```python
from build123d import *

# Parameters (mm, degrees)
SKETCH1_R           = 11
SKETCH1_R_2         = 2
SKETCH1_R_3         = 5
BOSS_EXTRUDE2_DEPTH = 5
BOSS_EXTRUDE4_DEPTH = 5
SKETCH2_W           = 50
SKETCH2_H           = 5
BOSS_EXTRUDE7_DEPTH = 45
CUT_EXTRUDE1_REACH  = 64.081
SKETCH3_R           = 3
FILLET1_R           = 10


with BuildPart() as part:
    # Sketch1 → Boss-Extrude2 (new body)
    with BuildSketch(Plane.XY):
        Circle(SKETCH1_R)
        with Locations((-8, 0)):
            Circle(SKETCH1_R_2, mode=Mode.SUBTRACT)
        with Locations((0, -8)):
            Circle(SKETCH1_R_2, mode=Mode.SUBTRACT)
        with Locations((8, 0)):
            Circle(SKETCH1_R_2, mode=Mode.SUBTRACT)
        with Locations((0, 8)):
            Circle(SKETCH1_R_2, mode=Mode.SUBTRACT)
        Circle(SKETCH1_R_3, mode=Mode.SUBTRACT)
    extrude(amount=BOSS_EXTRUDE2_DEPTH)

    # Sketch1_9 → Boss-Extrude4 (add)
    with BuildSketch(Plane.XY):
        with BuildLine():
            Line((-25, 16), (-25, 11))
            Line((-25, 11), (-15, 11))
            Line((-15, 11), (-11, 0))
            ThreePointArc((-11, 0), (0, 11), (11, 0))
            Line((11, 0), (15, 11))
            Line((15, 11), (25, 11))
            Line((25, 11), (25, 16))
            Line((25, 16), (-25, 16))
        make_face()
    extrude(amount=BOSS_EXTRUDE4_DEPTH)

    # Sketch2 → Boss-Extrude7 (add)
    with BuildSketch(Plane.XY.offset(5)):
        with Locations((0, 13.5)):
            Rectangle(SKETCH2_W, SKETCH2_H)
    extrude(amount=BOSS_EXTRUDE7_DEPTH)

    # Sketch3 → Cut-Extrude1 (cut, up to next)
    with BuildSketch(Plane(origin=(0, 16, 0), x_dir=(1, 0, 0), z_dir=(0, 1, 0)), mode=Mode.PRIVATE) as cut_extrude1_sk1:
        with Locations(Location((10, -35, 0), (0, 0, 270))):
            Circle(SKETCH3_R)
    cut_extrude1_tool1 = extrude(cut_extrude1_sk1.sketch, amount=-CUT_EXTRUDE1_REACH, mode=Mode.PRIVATE) & part.part
    # Sketch3 → Cut-Extrude1 (cut, up to next)
    with BuildSketch(Plane(origin=(0, 16, 0), x_dir=(1, 0, 0), z_dir=(0, 1, 0)), mode=Mode.PRIVATE) as cut_extrude1_sk2:
        with Locations(Location((-10, -35, 0), (0, 0, 270))):
            Circle(SKETCH3_R)
    cut_extrude1_tool2 = extrude(cut_extrude1_sk2.sketch, amount=-CUT_EXTRUDE1_REACH, mode=Mode.PRIVATE) & part.part
    # Sketch3 → Cut-Extrude1 (cut, up to next)
    with BuildSketch(Plane(origin=(0, 16, 0), x_dir=(1, 0, 0), z_dir=(0, 1, 0)), mode=Mode.PRIVATE) as cut_extrude1_sk3:
        with Locations(Location((-10, -15, 0), (0, 0, 270))):
            Circle(SKETCH3_R)
    cut_extrude1_tool3 = extrude(cut_extrude1_sk3.sketch, amount=-CUT_EXTRUDE1_REACH, mode=Mode.PRIVATE) & part.part
    # Sketch3 → Cut-Extrude1 (cut, up to next)
    with BuildSketch(Plane(origin=(0, 16, 0), x_dir=(1, 0, 0), z_dir=(0, 1, 0)), mode=Mode.PRIVATE) as cut_extrude1_sk4:
        with Locations(Location((10, -15, 0), (0, 0, 270))):
            Circle(SKETCH3_R)
    cut_extrude1_tool4 = extrude(cut_extrude1_sk4.sketch, amount=-CUT_EXTRUDE1_REACH, mode=Mode.PRIVATE) & part.part
    add(cut_extrude1_tool1.solids().sort_by_distance((10, 16, 35))[0], mode=Mode.SUBTRACT)
    add(cut_extrude1_tool2.solids().sort_by_distance((-10, 16, 35))[0], mode=Mode.SUBTRACT)
    add(cut_extrude1_tool3.solids().sort_by_distance((-10, 16, 15))[0], mode=Mode.SUBTRACT)
    add(cut_extrude1_tool4.solids().sort_by_distance((10, 16, 15))[0], mode=Mode.SUBTRACT)

    # Fillet1
    fillet1_edges = [part.edges().sort_by_distance(p)[0] for p in [
        (25, 13.5, 0),
        (25, 13.5, 50),
        (-25, 13.5, 0),
        (-25, 13.5, 50),
    ]]
    fillet(fillet1_edges, radius=FILLET1_R)


solid = part.part
```
CAD build for the part. Positions are in the model's coordinates, mm. A direction names the side the tool comes from. Coordinates: 2 decimals unless noted, no trailing zeros. Order: outer loops, then holes, each group sorted by start corner. A loop starts at its lowest first (then second) coordinate and runs counter-clockwise, first axis right, second up. Notation, with made-up numbers: M 75.25,2.5 L 124.25,2.5 A5 ccw 124.25,7.5 Z; hole C -35.75,57.5 d5. An arc over 180 degrees is marked long. Write each question's results on one line, items separated by ' | '. Start each with the question number.
Q1. Cut at A-A (z = 15). List the corners of the cut face in (x, y).
Q2. Drill centre lines: probe 1 along Y at (x, z) = (2, 7.5); probe 2 along Z at (x, y) = (8.5, 9.5). Where is each one in solid material? Low to high. Write a range as from..to.
Q3. Pull direction Y, two halves, no side cores. Call faces 3 (the cylindrical face through (-22.15, 13.46, 3.01)), 4 (the cylindrical face through (-1.08, -4.88, 2.46)), 5 (the cylindrical face through (6, 0, 2)), 6 (the flat face through (12.97, 5.42, 2.46)): +Y half, -Y half, draft (parallel to the pull), parting line (faces both ways), or undercut.
Q4. Cut at B-B (x = 0). List the corners of the cut face in (y, z).
Q5. Cut at C-C (y = 7). List the corners of the cut face in (x, z), then the cut area to 3 significant figures.
Q6. Which spindle directions (+Z, -Z, +X, -X, +Y, -Y) get a long thin tool onto all of the face, cutting with end or side? Do faces 1 (the flat face through (25, 13, 25)), 2 (the flat face through (-4, 5, 5)). Say none if no direction does.
Q7. Cut at D-D (y = -0.75). List the corners of the cut face in (x, z).
Q8. Flat gauge pins, fed straight in: P1, Ø5, axis at x = 10, z = 15, coming from the +Y side; P2, Ø5, axis at x = -8, y = 0, coming from the +Z side; P3, Ø10, axis at x = 3, z = 30.5, coming from the -Y side; P4, Ø4, axis at y = 0, z = 6.5, coming from the +X side. Where does each tip first touch, or does it go through?
Found:
1) outline: M -25,11 L -13,11 L -13,16 L -25,16 Z; M -7,11 L 7,11 L 7,16 L -7,16 Z; M 13,11 L 25,11 L 25,16 L 13,16 Z
2) probe 1: 11..16 | probe 2: 0..5
3) face 3: draft | face 4: undercut | face 5: undercut | face 6: -Y half
4) outline: M -11,0 L -10,0 L -10,5 L -11,5 Z; M -6,0 L -5,0 L -5,5 L -6,5 Z; M 5,0 L 6,0 L 6,5 L 5,5 Z; M 10,0 L 16,0 L 16,50 L 11,50 L 11,5 L 10,5 Z
5) outline: M -13.55,0 L -1.73,0 L -1.73,5 L -13.55,5 Z; M 1.73,0 L 13.55,0 L 13.55,5 L 1.73,5 Z | area: 118 mm²
6) face 1: +Z, -Z, +X, +Y, -Y | face 2: +Z, +X, -X, -Y
7) outline: M -10.97,0 L -9.85,0 L -9.85,5 L -10.97,5 Z; M -6.15,0 L -4.94,0 L -4.94,5 L -6.15,5 Z; M 4.94,0 L 6.15,0 L 6.15,5 L 4.94,5 Z; M 9.85,0 L 10.97,0 L 10.97,5 L 9.85,5 Z
8) P1: through | P2: z = 5 | P3: y = 11 | P4: x = 11.48
